```python
from build123d import *

# Parameters (mm, degrees)
SKETCH1_R           = 5
BOSS_EXTRUDE1_DEPTH = 42.5
BOSS_EXTRUDE2_START = -37.5
SKETCH1_3_R         = 5
BOSS_EXTRUDE2_DEPTH = 5
BOSS_EXTRUDE3_START = -37.5
SKETCH1_4_R         = 5
BOSS_EXTRUDE3_DEPTH = 25
BOSS_EXTRUDE4_START = -57.5
BOSS_EXTRUDE4_DEPTH = 5
BOSS_EXTRUDE5_START = -57.5
SKETCH1_6_R         = 5
BOSS_EXTRUDE5_DEPTH = 42.5


with BuildPart() as part:
    # Sketch1 → Boss-Extrude1 (new body)
    with BuildSketch(Plane(origin=(0, 0, 0), x_dir=(0, 0, -1), z_dir=(1, 0, 0))):
        Circle(SKETCH1_R)
    extrude(amount=-BOSS_EXTRUDE1_DEPTH)

    # Sketch1<3> → Boss-Extrude2 (add)
    with BuildSketch(Plane(origin=(0, 0, 0), x_dir=(0, 0, -1), z_dir=(1, 0, 0)).offset(BOSS_EXTRUDE2_START)):
        with BuildLine():
            ThreePointArc((5, 20), (0, 15), (-5, 20))
            Line((-5, 20), (-5, 0))
            ThreePointArc((-5, 0), (0, 5), (5, 0))
            Line((5, 0), (5, 20))
        make_face()
        with Locations((0, 20)):
            Circle(SKETCH1_3_R)
    extrude(amount=-BOSS_EXTRUDE2_DEPTH)

    # Sketch1<4> → Boss-Extrude3 (add)
    with BuildSketch(Plane(origin=(0, 0, 0), x_dir=(0, 0, -1), z_dir=(1, 0, 0)).offset(BOSS_EXTRUDE3_START)):
        with Locations((0, 20)):
            Circle(SKETCH1_4_R)
    extrude(amount=-BOSS_EXTRUDE3_DEPTH)

    # Sketch1<5> → Boss-Extrude4 (add)
    with BuildSketch(Plane(origin=(0, 0, 0), x_dir=(0, 0, -1), z_dir=(1, 0, 0)).offset(BOSS_EXTRUDE4_START)):
        with BuildLine():
            ThreePointArc((5, 20), (0, 15), (-5, 20))
            Line((-5, 20), (-5, 0))
            ThreePointArc((-5, 0), (0, 5), (5, 0))
            Line((5, 0), (5, 20))
        make_face()
    extrude(amount=-BOSS_EXTRUDE4_DEPTH)

    # Sketch1<6> → Boss-Extrude5 (add)
    with BuildSketch(Plane(origin=(0, 0, 0), x_dir=(0, 0, -1), z_dir=(1, 0, 0)).offset(BOSS_EXTRUDE5_START)):
        Circle(SKETCH1_6_R)
    extrude(amount=-BOSS_EXTRUDE5_DEPTH)


solid = part.part
```
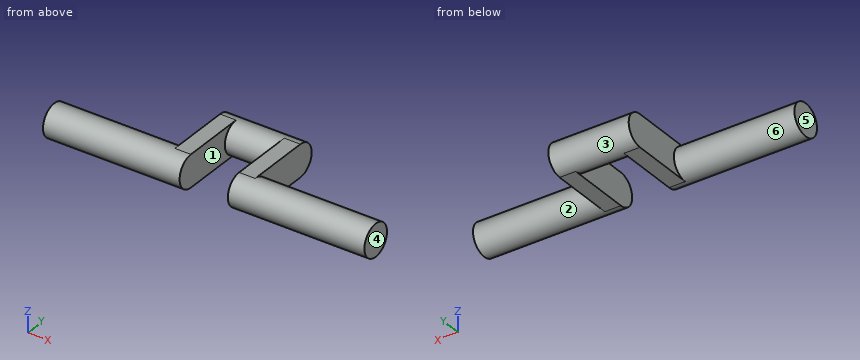
The listing builds one solid part. Answer for the finished solid, in the listing's coordinates (mm). Face numbers are marked on the shaded views. A direction names the side the tool comes from. Coordinates: 2 decimals unless noted, no trailing zeros. Loops run counter-clockwise (first coordinate to the right, second up) from the corner with the lowest first, then second, coordinate; pieces in that order, holes last. Notation, with made-up numbers: (-27.75, 62.25) -> (0.25, 62.25) arc R19 ccw to (0.25, 85.25) -> close; hole circle Ø11 at (-33.75, 4.5). An arc over 180 degrees is marked (long way). Use one line per item in the form item = value. Start each with the question number.
Item 1: A tool of negligible diameter and unlimited length cuts with its end or side. For the marked faces 5 and 6, from which of +Z, -Z, +X, -X, +Y, -Y can it reach the whole face along a straight path? Write none if from no direction.
Item 2: The part is cut by section A-A on y = 10.5. Determine the outline of the cut face in (x, z).
Item 3: The part is cut by section C-C on y = 16. Determine the outline of the cut face in (x, z).
Item 4: Flat-ended cylindrical pins translate along their axes: pin 1 Ø3 at (x, z) = (-22.5, -0.5) entering from +Y; pin 2 Ø5 at (x, z) = (-55.5, -4) entering from -Y. Find the tip coordinate at first contact, or state that the pin passes through.
Item 5: The mould has two halves that part along X. Classify the marked faces 1, 2, 3 and 4: released by +X, released by -X, zero draft, split by the parting line, or undercut.
Item 6: Consider L1, parallel to X at y = 5.5, z = 1; L2, parallel to X at y = 1.25, z = -4.25; L3, parallel to X at y = 21.25, z = 1.5. Determine where each line is inside the solid, lowest interval first. Write a range as [from, to].
Item 7: The part is cut by section B-B on z = -3. Determine the outline of the cut face in (x, y), then the cut area to 3 significant figures.
Item 8: The part is cut by section D-D on x = -65. Determine the outline of the cut face in (y, z).
Answer key:
q1.face_5 = +Z, -Z, -X, +Y, -Y
q1.face_6 = -X
q2.outline = (-62.5, -5) -> (-57.5, -5) -> (-57.5, 5) -> (-62.5, 5) -> close; (-42.5, -5) -> (-37.5, -5) -> (-37.5, 5) -> (-42.5, 5) -> close
q3.outline = (-62.5, -5) -> (-57.5, -5) -> (-57.5, -3) -> (-42.5, -3) -> (-42.5, -5) -> (-37.5, -5) -> (-37.5, 5) -> (-42.5, 5) -> (-42.5, 3) -> (-57.5, 3) -> (-57.5, 5) -> (-62.5, 5) -> close
q4.pin_1 = 5
q4.pin_2 = -4.33
q5.face_1 = undercut
q5.face_2 = zero draft
q5.face_3 = undercut
q5.face_4 = released by +X
q6.L1 = [-62.5, -57.5], [-42.5, -37.5]
q6.L2 = [-100, -57.5], [-42.5, 0]
q6.L3 = [-62.5, -37.5]
q7.outline = (-100, -4) -> (-57.5, -4) -> (-57.5, 16) -> (-42.5, 16) -> (-42.5, -4) -> (0, -4) -> (0, 4) -> (-37.5, 4) -> (-37.5, 24) -> (-62.5, 24) -> (-62.5, 4) -> (-100, 4) -> close
q7.area = 1,000 mm2
q8.outline = circle Ø10 at (0, 0)
